Read the model definition and answer for the solid it produces. Units are mm, in the model's axes. A direction names the side the tool comes from. Round coordinates to 2 decimals unless told otherwise and drop trailing zeros. Write each loop counter-clockwise with the first axis right and the second up, starting at its lowest first coordinate (ties: lowest second). Pieces come first, ordered by that corner, then holes. Notation, with made-up numbers: (-20, 68) - (-9, 68) arc R18 ccw to (-9, 91) - close; hole circle Ø7 at (33, 23). An arc over 180 degrees is marked (long way). One line per item, written item: value. Start each with the question number.
(1) For faces 1 (the face through (3, -3, 2.4)), 2 (the face through (-15, 0, 1)), 3 (the face through (3, 11, 0)), determine the directions among +Z, -Z, +X, -X, +Y, -Y from which every point of the face is accessible in a straight line to the end or side of a thin tool.
(2) Flat-ended cylindrical pins translate along their axes: pin 1 Ø10 at (y, z) = (-6.5, 3) entering from -X; pin 2 Ø3.5 at (x, y) = (13.5, 0) entering from -Z; pin 3 Ø6 at (y, z) = (8.5, -10.5) entering from -X. Find the tip coordinate at first contact, or state that the pin passes through.
(3) Find the intervals of material crossed by L1, parallel to Y at x = 0, z = 1.35; L2, parallel to Z at x = 3.5, y = -14; L3, parallel to Y at x = 0, z = 9.5, in increasing order.
(4) The mould has two halves that part along Y. Classify faces 4 (the face through (0, 0, -16.6)), 5 (the face through (12, 0, 1)), 6 (the face through (-3.47, -15.62, 1.18)): +Y half, -Y half, draft (parallel to the pull), parting line (faces both ways), or undercut.
(5) A cutting plane is placed at D-D, the plane x = -8. Determine the outline of the cut face in (y, z).
(6) A cutting plane is placed at B-B, the plane x = 0. Determine the outline of the cut face in (y, z).
(7) A cutting plane is placed at A-A, the plane z = 0.5. Determine the outline of the cut face in (x, y).
(8) A cutting plane is placed at C-C, the plane y = -13.5. Determine the outline of the cut face in (x, z), plus the area to 3 significant figures.
from build123d import *

# Parameters (mm, degrees)
SKETCH_1_R      = 16
SKETCH_1_R_2    = 1.5
EXTRUDE_1_DEPTH = 2.4
SKETCH_2_R      = 3.9
EXTRUDE_2_DEPTH = 9
SKETCH_3_R      = 11
EXTRUDE_3_DEPTH = 16.6


with BuildPart() as part:
    # Эскиз1 → Бобышка-Вытянуть1 (new body)
    with BuildSketch(Plane.XY):
        Circle(SKETCH_1_R)
        with Locations((-13.5, 0)):
            Circle(SKETCH_1_R_2, mode=Mode.SUBTRACT)
        with Locations((0, 13.5)):
            Circle(SKETCH_1_R_2, mode=Mode.SUBTRACT)
        with Locations((13.5, 0)):
            Circle(SKETCH_1_R_2, mode=Mode.SUBTRACT)
        with Locations((0, -13.5)):
            Circle(SKETCH_1_R_2, mode=Mode.SUBTRACT)
    extrude(amount=EXTRUDE_1_DEPTH)

    # Эскиз2 → Бобышка-Вытянуть2 (add)
    with BuildSketch(Plane.XY.offset(2.4)):
        Circle(SKETCH_2_R)
    extrude(amount=EXTRUDE_2_DEPTH)

    # Эскиз3 → Бобышка-Вытянуть3 (add)
    with BuildSketch(Plane(origin=(0, 0, 0), x_dir=(-1, 0, 0), z_dir=(0, 0, -1))):
        Circle(SKETCH_3_R)
    extrude(amount=EXTRUDE_3_DEPTH)


solid = part.part
Here are the results:
1. face 1: +Z
1. face 2: +Z, -Z
1. face 3: -Z
2. pin 1: x = -15.93
2. pin 2: z = 0
2. pin 3: x = -9.53
3. L1: -16 to -15, -12 to 12, 15 to 16
3. L2: 0 to 2.4
3. L3: -3.9 to 3.9
4. face 4: draft
4. face 5: undercut
4. face 6: parting line
5. outline: (-13.86, 0) - (-7.55, 0) - (-7.55, -16.6) - (7.55, -16.6) - (7.55, 0) - (13.86, 0) - (13.86, 2.4) - (-13.86, 2.4) - close
6. outline: (-16, 0) - (-15, 0) - (-15, 2.4) - (-16, 2.4) - close; (-12, 0) - (-11, 0) - (-11, -16.6) - (11, -16.6) - (11, 0) - (12, 0) - (12, 2.4) - (3.9, 2.4) - (3.9, 11.4) - (-3.9, 11.4) - (-3.9, 2.4) - (-12, 2.4) - close; (15, 0) - (16, 0) - (16, 2.4) - (15, 2.4) - close
7. outline: circle Ø32 at (0, 0); hole circle Ø3 at (-13.5, 0); hole circle Ø3 at (0, -13.5); hole circle Ø3 at (0, 13.5); hole circle Ø3 at (13.5, 0)
8. outline: (-8.59, 0) - (-1.5, 0) - (-1.5, 2.4) - (-8.59, 2.4) - close; (1.5, 0) - (8.59, 0) - (8.59, 2.4) - (1.5, 2.4) - close
8. area: 34.0 mm²
